Check sheet for the modelled part. Datum: model origin and axes. Units: mm. A direction names the side the tool comes from. Coordinates: 2 decimals unless noted, no trailing zeros. Order: outer loops, then holes, each group sorted by start corner. A loop starts at its lowest first (then second) coordinate and runs counter-clockwise, first axis right, second up.
1. Cross-section at A-A (x = -14). Enter the section's corners in (y, z).
2. Cross-section at C-C (z = -7.5). Enter the section's corners in (x, y), then the cut area to 3 significant figures.
3. Thickness scan on line 1 (Y direction, x = 0, z = 0.6); line 2 (Y direction, x = 0, z = -2.5); line 3 (Y direction, x = 0, z = -16.5). Record the ranges inside material, lowest first.
4. Set-up check for faces 4 (the cylindrical face through (1.487, -5.579, -20.795)), 5 (the cylindrical face through (7.493, 0.33, -12.049)), 6 (the flat face through (-4.3, 0.3, 3)): record each of +Z, -Z, +X, -X, +Y, -Y from which the full face is reachable in a straight line by a thin tool's end or side.
5. Gauge pin test, flat ends, axial feed: pin 1 Ø4 at (x, y) = (-14, 0) entering from -Z; pin 2 Ø10.5 at (x, y) = (0, 0) entering from -Z; pin 3 Ø6 at (x, z) = (0.5, -10.5) entering from +Y; pin 4 Ø3.5 at (y, z) = (0, -20.6) entering from -X. Record the tip position at first contact, or that the pin passes through.
6. Draft check along X on faces 1 (the cylindrical face through (-5.577, 1.487, -20.405)), 2 (the cylindrical face through (0.93, 7.09, -16.06)), 3 (the cylindrical face through (-15.5, 0.07, 1.48)). Enter one of: released by +X, released by -X, zero draft, split by the parting line, or undercut.
7. Cross-section at D-D (x = 0). Count the separate pieces of the cut face and the enclosed holes in it, then the cut area to 3 significant figures.
```python
from build123d import *
from build123d.topology import SkipClean

# Parameters (mm, degrees)
SKETCH_1_R               = 18
SKETCH_1_R_2             = 1.5
SKETCH_1_R_3             = 4
EXTRUDE_1_DEPTH          = 3
EXTRUDE_START            = 8.5
SKETCH_2_R               = 9
SKETCH_2_R_2             = 4
EXTRUDE_2_DEPTH          = 8.5
EXTRUDE_START_2          = 15
SKETCH_3_R               = 7.5
SKETCH_3_R_2             = 4
EXTRUDE_3_DEPTH          = 15
CUT_EXTRUDE_START        = 1.1
SKETCH_4_R               = 7.5
SKETCH_4_R_2             = 7.15
CUT_EXTRUDE_2_DEPTH      = 1.1
CUT_EXTRUDE_3_REACH      = 36.645
CUT_EXTRUDE_3_END_RADIUS = 7.5
SKETCH_5_R               = 1.5
CUT_EXTRUDE_4_REACH      = 36.645
CUT_EXTRUDE_4_END_RADIUS = 7.5
SKETCH_7_R               = 1.5


with BuildPart() as part:
    # 草图1 → 凸台-拉伸1 (new body)
    with BuildSketch(Plane.XY):
        Circle(SKETCH_1_R)
        with Locations((0, 14)):
            Circle(SKETCH_1_R_2, mode=Mode.SUBTRACT)
        with Locations((14, 0)):
            Circle(SKETCH_1_R_2, mode=Mode.SUBTRACT)
        with Locations((0, -14)):
            Circle(SKETCH_1_R_2, mode=Mode.SUBTRACT)
        with Locations((-14, 0)):
            Circle(SKETCH_1_R_2, mode=Mode.SUBTRACT)
        Circle(SKETCH_1_R_3, mode=Mode.SUBTRACT)
    extrude(amount=EXTRUDE_1_DEPTH)

    # 草图2 → 凸台-拉伸2 (add)
    with SkipClean():  # the faces are left unmerged after this step: merging them gives an invalid solid
        with BuildSketch(Plane(origin=(0, 0, 0), x_dir=(-1, 0, 0), z_dir=(0, 0, -1)).offset(EXTRUDE_START)):
            with Locations(Location((0, 0, 0), (0, 0, 180))):
                Circle(SKETCH_2_R)
            Circle(SKETCH_2_R_2, mode=Mode.SUBTRACT)
        extrude(amount=-EXTRUDE_2_DEPTH)

    # 草图3 → 凸台-拉伸3 (add)
    with SkipClean():  # the faces are left unmerged after this step: merging them gives an invalid solid
        with BuildSketch(Plane(origin=(0, 0, -8.5), x_dir=(-1, 0, 0), z_dir=(0, 0, -1)).offset(EXTRUDE_START_2)):
            Circle(SKETCH_3_R)
            Circle(SKETCH_3_R_2, mode=Mode.SUBTRACT)
        extrude(amount=-EXTRUDE_3_DEPTH)

    # 草图4 → 切除-拉伸2 (cut)
    with SkipClean():  # the faces are left unmerged after this step: merging them gives an invalid solid
        with BuildSketch(Plane(origin=(0, 0, -15.5), x_dir=(-1, 0, 0), z_dir=(0, 0, -1)).offset(CUT_EXTRUDE_START)):
            Circle(SKETCH_4_R)
            Circle(SKETCH_4_R_2, mode=Mode.SUBTRACT)
        extrude(amount=-CUT_EXTRUDE_2_DEPTH, mode=Mode.SUBTRACT)

    # 切除-拉伸3: up to this cylinder (the profile starts inside it)
    with SkipClean():  # the faces are left unmerged after this step: merging them gives an invalid solid
        cut_extrude_3_end = Plane(origin=(0, 0, -20.6), z_dir=(0, 0, 1)) * Cylinder(CUT_EXTRUDE_3_END_RADIUS, 89.29, mode=Mode.PRIVATE)
        # 草图5 → 切除-拉伸3 (cut, up to the surface)
        with BuildSketch(Plane(origin=(0, 0, 0), x_dir=(1, 0, 0), z_dir=(0, 1, 0)), mode=Mode.PRIVATE) as cut_extrude_3_sk1:
            with Locations(Location((0, 20.6, 0), (0, 0, 270))):
                Circle(SKETCH_5_R)
        cut_extrude_3_tool1 = extrude(cut_extrude_3_sk1.sketch, amount=-CUT_EXTRUDE_3_REACH, mode=Mode.PRIVATE) & cut_extrude_3_end
        add(cut_extrude_3_tool1.solids().sort_by_distance((0, 0, -20.6))[0], mode=Mode.SUBTRACT)

    # 切除-拉伸4: up to this cylinder (the profile starts inside it)
    with SkipClean():  # the faces are left unmerged after this step: merging them gives an invalid solid
        cut_extrude_4_end = Plane(origin=(0, 0, -20.6), z_dir=(0, 0, 1)) * Cylinder(CUT_EXTRUDE_4_END_RADIUS, 89.29, mode=Mode.PRIVATE)
        # 草图7 → 切除-拉伸4 (cut, up to the surface)
        with BuildSketch(Plane(origin=(0, 0, 0), x_dir=(0, 0, -1), z_dir=(1, 0, 0)), mode=Mode.PRIVATE) as cut_extrude_4_sk1:
            with Locations((20.6, 0)):
                Circle(SKETCH_7_R)
        cut_extrude_4_tool1 = extrude(cut_extrude_4_sk1.sketch, amount=-CUT_EXTRUDE_4_REACH, mode=Mode.PRIVATE) & cut_extrude_4_end
        add(cut_extrude_4_tool1.solids().sort_by_distance((0, 0, -20.6))[0], mode=Mode.SUBTRACT)


solid = part.part
```
Data:
1. outline: (-11.31, 0) - (-1.5, 0) - (-1.5, 3) - (-11.31, 3) - close; (1.5, 0) - (11.31, 0) - (11.31, 3) - (1.5, 3) - close
2. outline: circle Ø18 at (0, 0); hole circle Ø8 at (0, 0)
2. area: 204 mm2
3. line 1: y = -18 to -15.5, -12.5 to -4, 4 to 12.5, 15.5 to 18
3. line 2: y = -9 to -4, 4 to 9
3. line 3: y = -7.15 to -4, 4 to 7.15
4. face 4: -Y
4. face 5: -Z
4. face 6: +Z, +X, -X, +Y, -Y
5. pin 1: stops at z = 0
5. pin 2: stops at z = -23.5
5. pin 3: stops at y = 9
5. pin 4: stops at x = -7.5
6. face 1: zero draft
6. face 2: split by the parting line
6. face 3: undercut
7. separate pieces: 5
7. enclosed holes: 0
7. area: 245 mm2
